Read the model definition and answer for the solid it produces. Units are mm, in the model's axes. Face numbers are marked on the shaded views. A direction names the side the tool comes from. Coordinates: 2 decimals unless noted, no trailing zeros. Write each loop counter-clockwise with the first axis right and the second up, starting at its lowest first coordinate (ties: lowest second). Pieces come first, ordered by that corner, then holes.
(1) The part is cut by section B-B, the plane x = 0. Determine the outline of the cut face in (y, z), and give its area (3 significant figures).
(2) The part is cut by section C-C, the plane z = 11.5. Determine the outline of the cut face in (x, y), and give its area (3 significant figures).
(3) The part is cut by section D-D, the plane y = 84. Determine the outline of the cut face in (x, z), and give its area (3 significant figures).
(4) Which of the six approach directions +Z, -Z, +X, -X, +Y, -Y give full straight-line access (tool end or side, diameter ignored) to the marked faces 1 and 2?
(5) Determine the mould class of the marked faces 3, 4, 5 and 6 for opening direction X: pulls with the +X half, pulls with the -X half, needs draft (parallel to the pull), parting line crosses it, or undercut.
(6) The part is cut by section A-A, the plane z = 20. Determine the outline of the cut face in (x, y).
(7) Straight lines are drawn through the part: line 1 along Y through (x, z) = (-1.75, 27); line 2 along Z through (x, y) = (0, 4.6); line 3 along X through (y, z) = (64, 20). For each, find the intervals that lie inside material, in ascending order.
(8) Given pin 1 (10 mm diameter, centred on x = -2.5, y = 35.5, fed in from +Z); pin 2 (2.5 mm diameter, centred on x = 0, z = 20, fed in from -Y); pin 3 (3 mm diameter, centred on x = 5, y = 66, fed in from +Z); pin 4 (8 mm diameter, centred on x = -3.5, y = 74.5, fed in from -Z), each flat-ended and moving along its own axis, determine where each tip first touches the part or whether it passes through.
```python
from build123d import *

# Parameters (mm, degrees)
SKETCH1_W           = 22.1
SKETCH1_H           = 11.1
SKETCH1_W_2         = 18.1
SKETCH1_H_2         = 7.1
BOSS_EXTRUDE1_DEPTH = 40
SKETCH2_R           = 1.5
CUT_EXTRUDE1_DEPTH  = 33
SKETCH3_R           = 7.5
SKETCH3_R_2         = 6.5
BOSS_EXTRUDE3_DEPTH = 90


with BuildPart() as part:
    # Sketch1 → Boss-Extrude1 (new body)
    with BuildSketch(Plane.XY):
        Rectangle(SKETCH1_W, SKETCH1_H)
        Rectangle(SKETCH1_W_2, SKETCH1_H_2, mode=Mode.SUBTRACT)
    extrude(amount=BOSS_EXTRUDE1_DEPTH)

    # Sketch2 → Cut-Extrude1 (cut)
    with BuildSketch(Plane.XZ.offset(5.55)):
        with Locations((0, 20)):
            Circle(SKETCH2_R)
    extrude(amount=-CUT_EXTRUDE1_DEPTH, mode=Mode.SUBTRACT)

    # Sketch3 → Boss-Extrude3 (add)
    with BuildSketch(Plane(origin=(0, 5.55, 0), x_dir=(1, 0, 0), z_dir=(0, 1, 0))):
        with Locations((0, -20)):
            Circle(SKETCH3_R)
        with Locations((0, -20)):
            Circle(SKETCH3_R_2, mode=Mode.SUBTRACT)
    extrude(amount=BOSS_EXTRUDE3_DEPTH)


solid = part.part
```
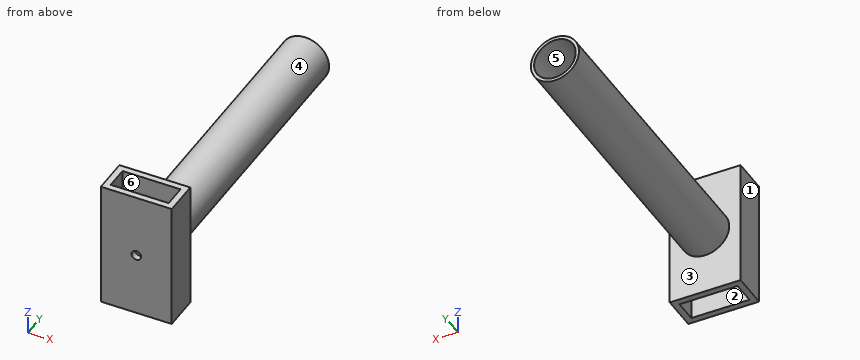
Computed:
1. outline: (-5.55, 0) - (-3.55, 0) - (-3.55, 18.5) - (-5.55, 18.5) - close; (-5.55, 21.5) - (-3.55, 21.5) - (-3.55, 40) - (-5.55, 40) - close; (3.55, 0) - (5.55, 0) - (5.55, 12.5) - (95.55, 12.5) - (95.55, 13.5) - (5.55, 13.5) - (5.55, 18.5) - (3.55, 18.5) - close; (3.55, 21.5) - (5.55, 21.5) - (5.55, 26.5) - (95.55, 26.5) - (95.55, 27.5) - (5.55, 27.5) - (5.55, 40) - (3.55, 40) - close
1. area: 328 mm2
2. outline: (-11.05, -5.55) - (11.05, -5.55) - (11.05, 5.55) - (-11.05, 5.55) - close; hole (-9.05, -3.55) - (9.05, -3.55) - (9.05, 3.55) - (-9.05, 3.55) - close
2. area: 117 mm2
3. outline: circle Ø15 at (0, 20); hole circle Ø13 at (0, 20)
3. area: 44.0 mm2
4. face 1: +Z, -Z, -X, +Y, -Y
4. face 2: +Z, -Z
5. face 3: needs draft
5. face 4: parting line crosses it
5. face 5: undercut
5. face 6: undercut
6. outline: (-11.05, -5.55) - (-1.5, -5.55) - (-1.5, -3.55) - (-9.05, -3.55) - (-9.05, 3.55) - (-1.5, 3.55) - (-1.5, 5.55) - (-6.5, 5.55) - (-6.5, 95.55) - (-7.5, 95.55) - (-7.5, 5.55) - (-11.05, 5.55) - close; (1.5, -5.55) - (11.05, -5.55) - (11.05, 5.55) - (7.5, 5.55) - (7.5, 95.55) - (6.5, 95.55) - (6.5, 5.55) - (1.5, 5.55) - (1.5, 3.55) - (9.05, 3.55) - (9.05, -3.55) - (1.5, -3.55) - close
7. line 1: y = -5.55 to -3.55, 3.55 to 95.55
7. line 2: z = 0 to 18.5, 21.5 to 40
7. line 3: x = -7.5 to -6.5, 6.5 to 7.5
8. pin 1: stops at z = 27.5
8. pin 2: passes through
8. pin 3: stops at z = 26.63
8. pin 4: stops at z = 12.5
